```python
from build123d import *

# Parameters (mm, degrees)
F0_R     = 15.875
F0_R_2   = 2.54
F1_DEPTH = 1.5875
F2_R     = 15.875
F2_R_2   = 10.795
F3_DEPTH = 4.7625
F4_SIZE  = 0.508


with BuildPart() as f1:
    # F0 (on Top) → F1 (new body)
    with BuildSketch(Plane.XY):
        Circle(F0_R)
        Circle(F0_R_2, mode=Mode.SUBTRACT)
    extrude(amount=F1_DEPTH)

    # F2 (on face) → F3 (join)
    with BuildSketch(Plane.XY.offset(1.5875)):
        Circle(F2_R)
        Circle(F2_R_2, mode=Mode.SUBTRACT)
    extrude(amount=F3_DEPTH)

    # F4
    f4_edges = [f1.edges().sort_by_distance(p)[0] for p in [
        (-10.795, 0, 6.35),
        (-2.54, 0, 1.5875),
    ]]
    chamfer(f4_edges, length=F4_SIZE)


solid = f1.part
```
Geometry check sheet. Reference: the model listing, model coordinates, mm. A direction names the side the tool comes from. Give positions to 0.01 mm unless a question says otherwise; leave off trailing zeros. Loops run counter-clockwise (first coordinate to the right, second up) from the corner with the lowest first, then second, coordinate; pieces in that order, holes last. Notation, with made-up numbers: M -6.75,60.25 L 48.25,60.25 A20 ccw 48.25,84.25 Z; hole C 41.25,85 d11. An arc over 180 degrees is marked long. Write item = value, one per line. Start each with the question number.
1. Section check C-C, the plane z = 5.25. Enter the section's corners in (x, y) (3 decimals), plus the area to 3 significant figures.
2. Section check D-D, the plane y = -12. Enter the section's corners in (x, z).
3. Go/stop test with flat-tipped pins: P1, Ø1, axis at x = -8.5, z = 1, coming from the -Y side; P2, Ø3, axis at y = -3.5, z = 3, coming from the -X side; P3, Ø4.5, axis at x = 0, y = 0, coming from the -Z side; P4, Ø2, axis at x = -3, z = 2.5, coming from the +Y side. Record where each tip stops, or that it passes through.
4. Draft check along Y on faces 1 (the face through (-3, -2, 1.588)), 2 (the face through (-4, 11, 6.35)), 3 (the face through (-3.441, -15.497, 3.131)). Enter one of: +Y half, -Y half, draft (parallel to the pull), parting line (faces both ways), or undercut.
5. Tool access check on faces 4 (the face through (3, 0, 0)), 5 (the face through (-7.956, 7.296, 3.685)). Record the directions out of +Z, -Z, +X, -X, +Y, -Y that give a thin tool (end or side, any length) a straight path to the whole face; none if there is none.
6. Thickness scan on probe 1 along Y at (x, z) = (0, 0.35) (3 decimals); probe 2 along Z at (x, y) = (-9, -4); probe 3 along Y at (x, z) = (3, 3.5). Record the ranges inside material, lowest first.
Values follow:
q1.outline = C 0,0 d31.75; hole C 0,0 d21.59
q1.area = 426 mm^2
q2.outline = M -10.39,0 L 10.39,0 L 10.39,6.35 L -10.39,6.35 Z
q3.P1 = -13.71
q3.P2 = -15.75
q3.P3 = through
q3.P4 = 15.75
q4.face_1 = undercut
q4.face_2 = draft
q4.face_3 = parting line
q5.face_4 = -Z, +X, -X, +Y, -Y
q5.face_5 = +Z
q6.probe_1 = -15.875 to -2.54, 2.54 to 15.875
q6.probe_2 = 0 to 1.59
q6.probe_3 = -15.59 to -10.37, 10.37 to 15.59
